The listing builds one solid part. Answer for the finished solid, in the listing's coordinates (mm). A direction names the side the tool comes from. Give positions to 0.01 mm unless a question says otherwise; leave off trailing zeros. Order: outer loops, then holes, each group sorted by start corner. A loop starts at its lowest first (then second) coordinate and runs counter-clockwise, first axis right, second up. Notation, with made-up numbers: (30, 24.5) - (75, 24.5) arc R19 ccw to (75, 56.5) - close; hole circle Ø10 at (87, -29). An arc over 180 degrees is marked (long way). Write each question's results on one line, items separated by ' | '. Start each with the question number.
1. Section C-C (x = 321) is taken. Give the vertices of the cut face in (y, z), and give its area (3 significant figures).
2. Section D-D (x = 329.3) is taken. Give the vertices of the cut face in (y, z).
3. Determine the mould class of faces 4 (the face through (329, 283, 280.3)), 5 (the face through (291, 293, 280)) for opening direction X: released by +X, released by -X, zero draft, split by the parting line, or undercut.
4. Section B-B (y = 300) is taken. Give the vertices of the cut face in (x, z).
5. Section A-A (z = 285.75) is taken. Give the vertices of the cut face in (x, y), and give its area (3 significant figures).
6. Find the intervals of material crossed by L1, parallel to Y at x = 300, z = 282; L2, parallel to X at y = 283, z = 282.5; L3, parallel to X at y = 277.5, z = 281.8, in increasing order.
7. Which of the six approach directions +Z, -Z, +X, -X, +Y, -Y give full straight-line access (tool end or side, diameter ignored) to faces 1 (the face through (327.5, 276, 286)), 2 (the face through (271, 283, 280.3)), 3 (the face through (272.5, 324, 286))?
8. Flat-ended cylindrical pins translate along their axes: pin 1 (3 mm diameter, centred on x = 293.5, y = 293.5, fed in from +Z); pin 2 (1 mm diameter, centred on x = 333.5, z = 286.5, fed in from -Y); pin 3 (3.5 mm diameter, centred on x = 329.3, y = 317, fed in from +Z). Find the tip coordinate at first contact, or state that the pin passes through.
from build123d import *

# Parameters (mm, degrees)
SKETCH1_W           = 72
SKETCH1_H           = 58.3
SKETCH1_R           = 10
SKETCH1_R_2         = 1.45
BOSS_EXTRUDE1_DEPTH = 5
SKETCH2_W           = 8.5
SKETCH2_H           = 52
BOSS_EXTRUDE2_DEPTH = 7
SKETCH3_R           = 5.05
BOSS_EXTRUDE3_DEPTH = 7
SKETCH4_R           = 5.05
BOSS_EXTRUDE4_DEPTH = 7
SKETCH5_R           = 2.05
CUT_EXTRUDE1_DEPTH  = 6.7
SKETCH6_W           = 8.5
SKETCH6_H           = 52
BOSS_EXTRUDE5_DEPTH = 7
SKETCH7_R           = 5.05
BOSS_EXTRUDE6_DEPTH = 7
SKETCH8_R           = 5.05
BOSS_EXTRUDE7_DEPTH = 7
SKETCH9_R           = 2.05
CUT_EXTRUDE2_DEPTH  = 6.7


with BuildPart() as part:
    # Sketch1 → Boss-Extrude1 (new body)
    with BuildSketch(Plane.XY.offset(280)):
        with Locations((300, 299.15)):
            Rectangle(SKETCH1_W, SKETCH1_H)
        with Locations((300, 300)):
            Circle(SKETCH1_R, mode=Mode.SUBTRACT)
        with Locations((286.774831823, 318.202882373)):
            Circle(SKETCH1_R_2, mode=Mode.SUBTRACT)
        with Locations((278.601228383, 293.047117627)):
            Circle(SKETCH1_R_2, mode=Mode.SUBTRACT)
        with Locations((300, 277.5)):
            Circle(SKETCH1_R_2, mode=Mode.SUBTRACT)
        with Locations((321.398771617, 293.047117627)):
            Circle(SKETCH1_R_2, mode=Mode.SUBTRACT)
        with Locations((313.225168177, 318.202882373)):
            Circle(SKETCH1_R_2, mode=Mode.SUBTRACT)
    extrude(amount=BOSS_EXTRUDE1_DEPTH)

    # Sketch2 → Boss-Extrude2 (add)
    with BuildSketch(Plane.XY.offset(280)):
        with Locations((268.25, 300)):
            Rectangle(SKETCH2_W, SKETCH2_H)
    extrude(amount=BOSS_EXTRUDE2_DEPTH)

    # Sketch3 → Boss-Extrude3 (add)
    with BuildSketch(Plane.XY.offset(280)):
        with Locations((270.7, 283)):
            Circle(SKETCH3_R)
    extrude(amount=BOSS_EXTRUDE3_DEPTH)

    # Sketch4 → Boss-Extrude4 (add)
    with BuildSketch(Plane.XY.offset(280)):
        with Locations((270.7, 317)):
            Circle(SKETCH4_R)
    extrude(amount=BOSS_EXTRUDE4_DEPTH)

    # Sketch5 → Cut-Extrude1 (cut)
    with BuildSketch(Plane.XY.offset(280.3)):
        with Locations(Location((270.7, 283, 0), (0, 0, 180))):
            Circle(SKETCH5_R)
        with Locations(Location((270.7, 317, 0), (0, 0, 180))):
            Circle(SKETCH5_R)
    extrude(amount=CUT_EXTRUDE1_DEPTH, mode=Mode.SUBTRACT)

    # Sketch6 → Boss-Extrude5 (add)
    with BuildSketch(Plane.XY.offset(280)):
        with Locations((331.75, 300)):
            Rectangle(SKETCH6_W, SKETCH6_H)
    extrude(amount=BOSS_EXTRUDE5_DEPTH)

    # Sketch7 → Boss-Extrude6 (add)
    with BuildSketch(Plane.XY.offset(280)):
        with Locations((329.3, 283)):
            Circle(SKETCH7_R)
    extrude(amount=BOSS_EXTRUDE6_DEPTH)

    # Sketch8 → Boss-Extrude7 (add)
    with BuildSketch(Plane.XY.offset(280)):
        with Locations((329.3, 317)):
            Circle(SKETCH8_R)
    extrude(amount=BOSS_EXTRUDE7_DEPTH)

    # Sketch9 → Cut-Extrude2 (cut)
    with BuildSketch(Plane.XY.offset(280.3)):
        with Locations(Location((329.3, 283, 0), (0, 0, 180))):
            Circle(SKETCH9_R)
        with Locations(Location((329.3, 317, 0), (0, 0, 180))):
            Circle(SKETCH9_R)
    extrude(amount=CUT_EXTRUDE2_DEPTH, mode=Mode.SUBTRACT)


solid = part.part
Reported:
1) outline: (270, 280) - (291.65, 280) - (291.65, 285) - (270, 285) - close; (294.44, 280) - (328.3, 280) - (328.3, 285) - (294.44, 285) - close | area: 278 mm²
2) outline: (270, 280) - (328.3, 280) - (328.3, 285) - (326, 285) - (326, 287) - (319.05, 287) - (319.05, 280.3) - (314.95, 280.3) - (314.95, 287) - (285.05, 287) - (285.05, 280.3) - (280.95, 280.3) - (280.95, 287) - (274, 287) - (274, 285) - (270, 285) - close
3) face 4: undercut | face 5: zero draft
4) outline: (264, 280) - (290, 280) - (290, 285) - (272.5, 285) - (272.5, 287) - (264, 287) - close; (310, 280) - (336, 280) - (336, 287) - (327.5, 287) - (327.5, 285) - (310, 285) - close
5) outline: (264, 274) - (272.5, 274) - (272.5, 278.28) arc R5.05 ccw to (272.5, 287.72) - (272.5, 312.28) arc R5.05 ccw to (272.5, 321.72) - (272.5, 326) - (264, 326) - close; (327.5, 274) - (336, 274) - (336, 326) - (327.5, 326) - (327.5, 321.72) arc R5.05 ccw to (327.5, 312.28) - (327.5, 287.72) arc R5.05 ccw to (327.5, 278.28) - close; hole circle Ø4.1 at (270.7, 283); hole circle Ø4.1 at (270.7, 317); hole circle Ø4.1 at (329.3, 283); hole circle Ø4.1 at (329.3, 317) | area: 920 mm²
6) L1: 270 to 276.05, 278.95 to 290, 310 to 328.3 | L2: 264 to 268.65, 272.75 to 327.25, 331.35 to 336 | L3: 264 to 298.55, 301.45 to 336
7) face 1: +Z, -Y | face 2: +Z | face 3: +Z, +Y
8) pin 1: z = 285 | pin 2: y = 274 | pin 3: z = 280.3
